Source: three-view drawing plus pictorial views. Frame: mm from the lowest corner of the part. Give positions to 0.01 mm unless a question says otherwise; leave off trailing zeros. Loops run counter-clockwise (first coordinate to the right, second up) from the corner with the lowest first, then second, coordinate; pieces in that order, holes last. Notation, with made-up numbers: (-9, 9) - (31, 9) arc R26 cw to (31, 47) - close; hole circle Ø3 at (-11, -17.5). An arc over 180 degrees is marked (long way). Answer in a Markdown table with one row per item.
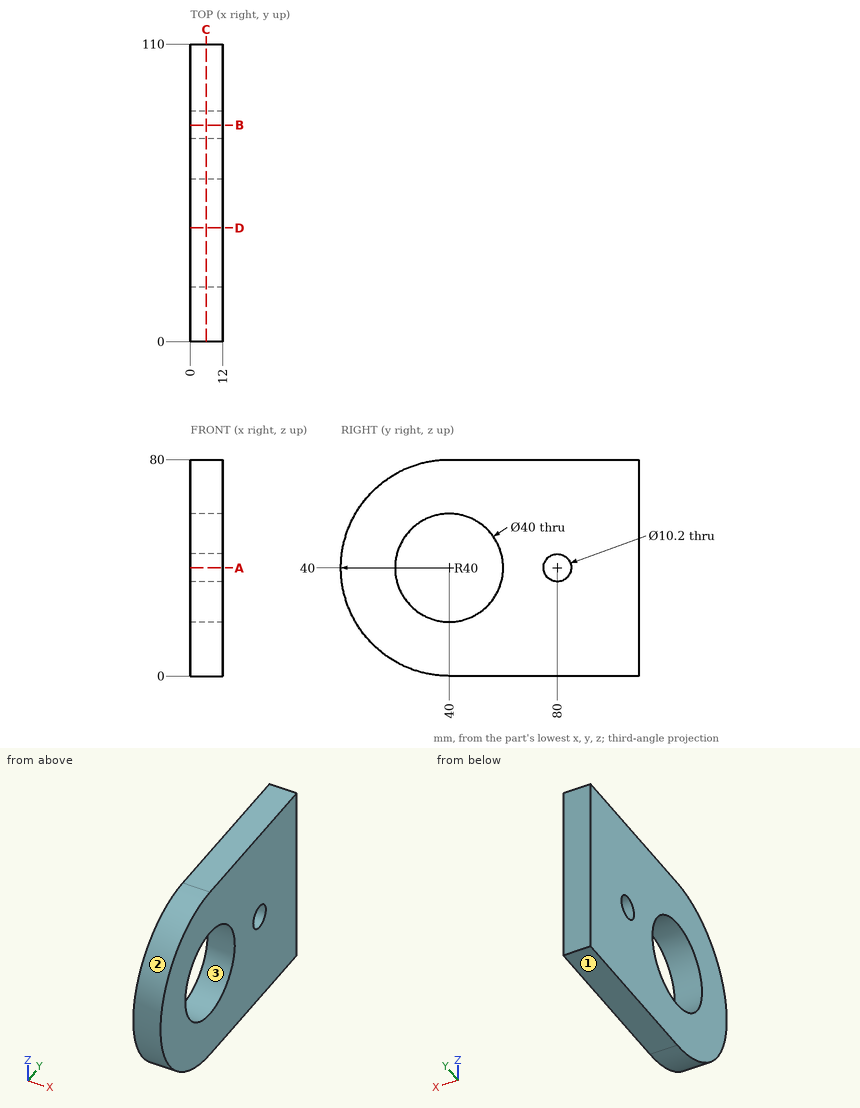
Q1. Draft query along Y for the marked faces 1, 2 and 3. Return one class per face: pulls with the +Y half, pulls with the -Y half, needs draft (parallel to the pull), parting line crosses it, or undercut.
Check values:
| item | result |
|---|---|
| face 1 | needs draft |
| face 2 | pulls with the -Y half |
| face 3 | undercut |
Q2. Cut plane C-C (x = 5.75). Output: boundary loops of the cut face in (y, z), and give its area (3 significant figures).
Check values:
| item | result |
|---|---|
| outline | (40, 0) - (110, 0) - (110, 80) - (40, 80) arc R40 ccw to start; hole circle Ø40 at (40, 40); hole circle Ø10.2 at (80, 40) |
| area | 6,770 mm² |
Q3. Cut plane B-B (y = 80). Output: boundary loops of the cut face in (x, z), and give its area (3 significant figures).
Check values:
| item | result |
|---|---|
| outline | (0, 0) - (12, 0) - (12, 34.9) - (0, 34.9) - close; (0, 45.1) - (12, 45.1) - (12, 80) - (0, 80) - close |
| area | 838 mm² |
Q4. Material intervals for line 1 along Y through (x, z) = (4.25, 40); line 2 along Z through (x, y) = (5.5, 21.5); line 3 along Z through (x, y) = (10.25, 31.5), sorted ascending.
Check values:
| item | result |
|---|---|
| line 1 | 0 to 20, 60 to 74.9, 85.1 to 110 |
| line 2 | 4.54 to 32.4, 47.6 to 75.46 |
| line 3 | 0.91 to 21.9, 58.1 to 79.09 |
Q5. Cut plane D-D (y = 42). Output: boundary loops of the cut face in (x, z), and give its area (3 significant figures).
Check values:
| item | result |
|---|---|
| outline | (0, 0) - (12, 0) - (12, 20.1) - (0, 20.1) - close; (0, 59.9) - (12, 59.9) - (12, 80) - (0, 80) - close |
| area | 482 mm² |
Q6. First-contact query: pin 1 (1.5 mm diameter, centred on x = 7, y = 29, fed in from -Z); pin 2 (2 mm diameter, centred on x = 6.5, y = 37, fed in from -Z); pin 3 (1 mm diameter, centred on x = 9, y = 34.5, fed in from -Z); pin 4 (9 mm diameter, centred on y = 80, z = 40, fed in from -X). Flat tips, straight axial feed; report the tip coordinate or a pass-through.
Check values:
| item | result |
|---|---|
| pin 1 | z = 1.34 |
| pin 2 | z = 0.05 |
| pin 3 | z = 0.31 |
| pin 4 | through |
Q7. Cut plane A-A (z = 40). Output: boundary loops of the cut face in (x, y), and give its area (3 significant figures).
Check values:
| item | result |
|---|---|
| outline | (0, 0) - (12, 0) - (12, 20) - (0, 20) - close; (0, 60) - (12, 60) - (12, 74.9) - (0, 74.9) - close; (0, 85.1) - (12, 85.1) - (12, 110) - (0, 110) - close |
| area | 718 mm² |
